```python
from build123d import *

# Parameters (mm, degrees)
F1_W     = 3.81
F1_H     = 1.905
F0_R     = 1.651
F3_DEPTH = 1.984375
F4_DEPTH = 6.35
F6_DEPTH = 0.79375


with BuildPart() as f2:
    # F1 (on Front) → F2 (revolve)
    with BuildSketch(Plane.XZ):
        with BuildLine():
            Line((3.81, 1.905), (3.81, 0))
            Line((3.81, 0), (5.3975, 0))
            ThreePointArc((5.3975, 0), (3.321495258, 2.7086744896), (0, 3.4925))
            Line((0, 3.4925), (0, 1.905))
            Line((0, 1.905), (3.81, 1.905))
        make_face()
        with Locations((1.905, 0.9525)):
            Rectangle(F1_W, F1_H)
    revolve(axis=Axis((0, 0, 2.69875), (0, 0, 1)))

    # F0 (on Top) → F3 (cut)
    with BuildSketch(Plane.XY):
        Polygon((1.8330871047, 3.175), (-1.8330871047, 3.175), (-3.6661742094, 0), (-1.8330871047, -3.175), (1.8330871047, -3.175), (3.6661742094, 0), align=None)
        Circle(F0_R, mode=Mode.SUBTRACT)
    extrude(amount=F3_DEPTH, mode=Mode.SUBTRACT)

    # F0 (on Top) → F4 (cut)
    with BuildSketch(Plane.XY):
        Circle(F0_R)
    extrude(amount=F4_DEPTH, mode=Mode.SUBTRACT)

    # F5 (on Front) → F6 (join, symmetric)
    with BuildSketch(Plane.XZ):
        Polygon((-5.3975, 0), (-3.81, 0), (-3.81, 1.5875), (-4.7399359697, 1.5875), (-8.1767540674, 5.0243180977), (-9.2992860825, 3.9017860825), align=None)
        with BuildLine():
            ThreePointArc((-8.1767540674, 5.0243180977), (-9.2992860825, 5.0243180977), (-9.2992860825, 3.9017860825))
            Line((-9.2992860825, 3.9017860825), (-8.1767540674, 5.0243180977))
        make_face()
        Polygon((3.81, 1.5875), (3.81, 0), (5.3975, 0), (9.2992860825, 3.9017860825), (8.1767540674, 5.0243180977), (4.7399359697, 1.5875), align=None)
        with BuildLine():
            Line((8.1767540674, 5.0243180977), (9.2992860825, 3.9017860825))
            ThreePointArc((9.2992860825, 3.9017860825), (9.2992860825, 5.0243180977), (8.1767540674, 5.0243180977))
        make_face()
    extrude(amount=F6_DEPTH, both=True)


solid = f2.part
```
The listing builds one solid part. Answer for the finished solid, in the listing's coordinates (mm). A direction names the side the tool comes from. Coordinates: 2 decimals unless noted, no trailing zeros. Loops run counter-clockwise (first coordinate to the right, second up) from the corner with the lowest first, then second, coordinate; pieces in that order, holes last. Notation, with made-up numbers: (-4.75, 43) -> (2.25, 43) arc R31 cw to (2.25, 67) -> close; hole circle Ø9 at (9.5, -20). An arc over 180 degrees is marked (long way). Use one line per item in the form item = value. Start each with the question number.
Item 1: Flat-ended cylindrical pins translate along their axes: pin 1 Ø1.6 at (x, z) = (-0.5, 1) entering from -Y; pin 2 Ø0.6 at (x, z) = (1, 1) entering from +Y; pin 3 Ø1.5 at (y, z) = (1, 2) entering from -X; pin 4 Ø3 at (x, y) = (0, 0) entering from -Z. Find the tip coordinate at first contact, or state that the pin passes through.
Item 2: The part is cut by section A-A on z = 4.2. Determine the outline of the cut face in (x, y).
Item 3: A tool of negligible diameter and unlimited length cuts with its end or side. For faces 1 (the face through (1.525, -0.632, 2.685)), 2 (the face through (-2.737, 1.61, 0.978)), 3 (the face through (-6.43, 0.01, 3.28)), from which of +Z, -Z, +X, -X, +Y, -Y can it reach the whole face along a straight path? Write none if from no direction.
Item 4: The part is cut by section B-B on x = 6.25. Determine the outline of the cut face in (y, z).
Item 5: The mould has two halves that part along X. Classify faces 4 (the face through (7.3, 0, 1.9)), 5 (the face through (2.76, 1.57, 0.98)), 6 (the face through (-7, -0.794, 3)), 7 (the face through (6.48, -0.01, 3.33)): released by +X, released by -X, zero draft, split by the parting line, or undercut.
Item 6: Consider L1, parallel to X at y = 0, z = 3.05; L2, parallel to X at y = 0, z = 2.85; L3, parallel to Y at x = 7.25, z = 2.6. Determine where each line is inside the solid, lowest interval first. Write a range as [from, to].
Answer key:
q1.pin_1 = -5.31
q1.pin_2 = 5.02
q1.pin_3 = -8.12
q1.pin_4 = through
q2.outline = (-9.49, -0.79) -> (-7.35, -0.79) -> (-7.35, 0.79) -> (-9.49, 0.79) -> close; (7.35, -0.79) -> (9.49, -0.79) -> (9.49, 0.79) -> (7.35, 0.79) -> close
q3.face_1 = +Z, -Z
q3.face_2 = -Z
q3.face_3 = +Z, +Y, -Y
q4.outline = (-0.79, 0.85) -> (0.79, 0.85) -> (0.79, 3.1) -> (-0.79, 3.1) -> close
q5.face_4 = released by +X
q5.face_5 = undercut
q5.face_6 = zero draft
q5.face_7 = undercut
q6.L1 = [-8.45, -6.2], [-2.7, -1.65], [1.65, 2.7], [6.2, 8.45]
q6.L2 = [-8.25, -6], [-3.09, -1.65], [1.65, 3.09], [6, 8.25]
q6.L3 = [-0.79, 0.79]
